Design review of the part shown in the three views and the two pictorial views. Dimensions are in mm from the part's minimum x, y and z. Round coordinates to 2 decimals unless told otherwise and drop trailing zeros. Loops run counter-clockwise (first coordinate to the right, second up) from the corner with the lowest first, then second, coordinate; pieces in that order, holes last. Notation, with made-up numbers: (17, 89) -> (36, 89) arc R30 ccw to (36, 113) -> close; hole circle Ø7 at (75.25, 59). An arc over 180 degrees is marked (long way). Use a Markdown table: item, result. Add a question column.
1) Consider section C-C on z = 45. Give the boundary of the cut face in (x, y) (1 decimal).
2) Consider section A-A on x = 67. Give the boundary of the cut face in (y, z) (1 decimal), plus the area to 3 significant figures.
3) Consider section B-B on y = 56. Give the boundary of the cut face in (x, z), plus the area to 3 significant figures.
4) Insertion check: pin 1 (2 mm diameter, centred on x = 55.5, z = 67, fed in from -Y); pin 2 (12 mm diameter, centred on y = 17, z = 58, fed in from +X); pin 3 (1.5 mm diameter, centred on y = 61, z = 33, fed in from +X). Each pin has a flat end and moves straight along its axis. Give the tip position at first contact, or say it passes through.
5) Wall thickness on probe 1 along Z at (x, y) = (105.5, 18); probe 2 along X at (y, z) = (52.5, 41) (1 decimal); probe 3 along Y at (x, z) = (38, 35) (1 decimal): over which ranges is each line inside the solid? List them lowest first.
6) Consider section D-D on y = 43. Give the boundary of the cut face in (x, z).
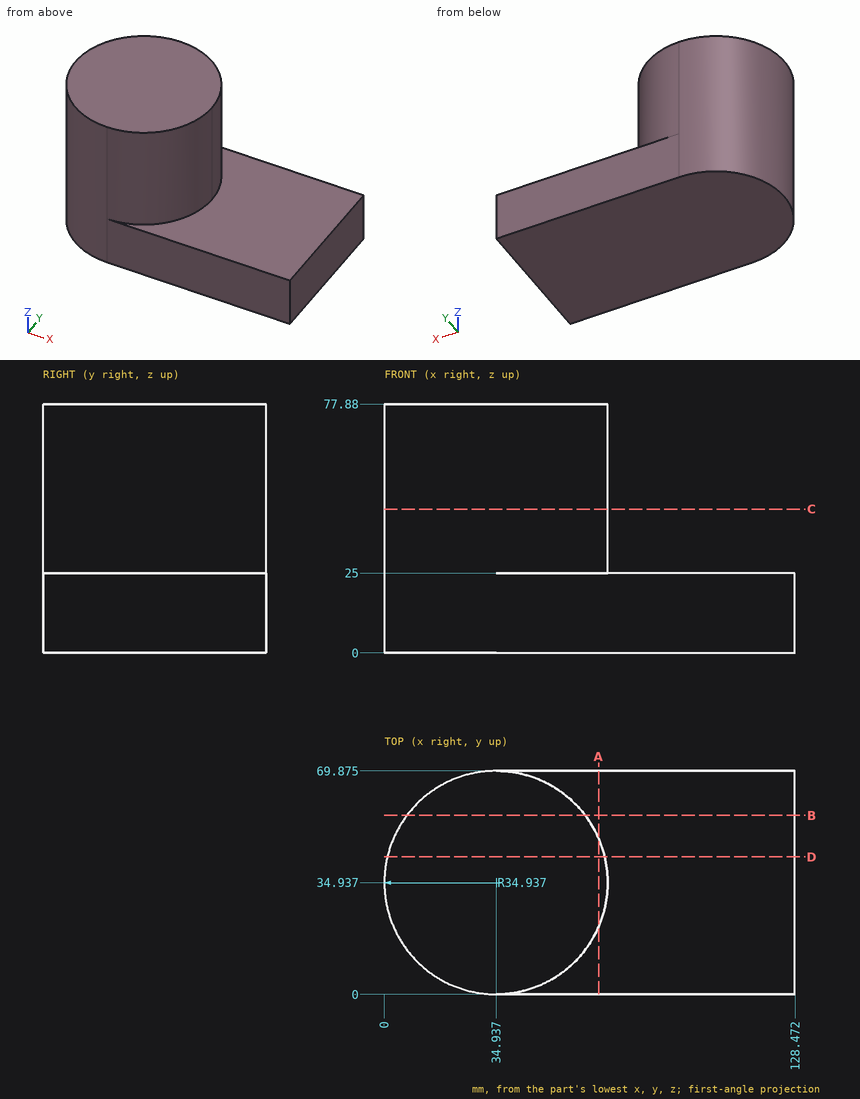
Result set:
| question | item | result |
|---|---|---|
| 1 | outline | (34.9, 0) arc R34.9 ccw to (69.9, 34.9) arc R34.9 ccw (long way) to start |
| 2 | outline | (0, 0) -> (69.9, 0) -> (69.9, 25) -> (48.8, 25) -> (48.8, 77.9) -> (21.1, 77.9) -> (21.1, 25) -> (0, 25) -> close |
| 2 | area | 3,210 mm2 |
| 3 | outline | (7.06, 0) -> (128.47, 0) -> (128.47, 25) -> (62.81, 25) -> (62.81, 77.88) -> (7.06, 77.88) -> close |
| 3 | area | 5,980 mm2 |
| 4 | pin 1 | y = 5.99 |
| 4 | pin 2 | x = 67.77 |
| 4 | pin 3 | x = 59.02 |
| 5 | probe 1 | 0 to 25 |
| 5 | probe 2 | 4.7 to 65.1 |
| 5 | probe 3 | 0.1 to 69.7 |
| 6 | outline | (0.94, 0) -> (128.47, 0) -> (128.47, 25) -> (68.93, 25) -> (68.93, 77.88) -> (0.94, 77.88) -> close |
